Design review of the part shown in the three views and the two pictorial views. Dimensions are in mm from the part's minimum x, y and z. A direction names the side the tool comes from. Round coordinates to 2 decimals unless told otherwise and drop trailing zeros. Loops run counter-clockwise (first coordinate to the right, second up) from the corner with the lowest first, then second, coordinate; pieces in that order, holes last.
1. Consider section A-A on x = 15.53. State the section outline as (y, z) points (1 decimal).
2. Clearance check with flat-ended pins moving along their axes: pin 1 Ø4 at (y, z) = (45.5, 5) entering from -X; pin 2 Ø3 at (y, z) = (77, 1.5) entering from +X; pin 3 Ø7 at (x, y) = (80.482, 66.756) entering from -Z; pin 4 Ø1 at (y, z) = (75.5, 7) entering from +X (1 decimal). State where each tip first meets the part, or that it passes through.
3. To check wall thickness, follow line 1 along Y through (x, z) = (79.5, 5.25) (1 decimal); line 2 along X through (y, z) = (69, 7.5) (1 decimal); line 3 along X through (y, z) = (31.5, 5.75) (1 decimal). State the ranges of each line that lie inside material, in increasing order.
4. Consider section B-B on z = 4.25. State how many separate pieces and enclosed holes the cut face has, then the cut area to 3 significant figures.
5. Tool access review of the marked faces 1 and 2: name each direction out of +Z, -Z, +X, -X, +Y, -Y from which nothing blocks a thin tool from reaching the whole face with its end or side.
6. Draft analysis for pull direction Y (two halves, no side actions). For the marked faces 3, 4 and 5, state which applies: released by +Y, released by -Y, zero draft, split by the parting line, or undercut.
7. Consider section D-D on y = 23.5. State the section outline as (x, z) points (1 decimal).
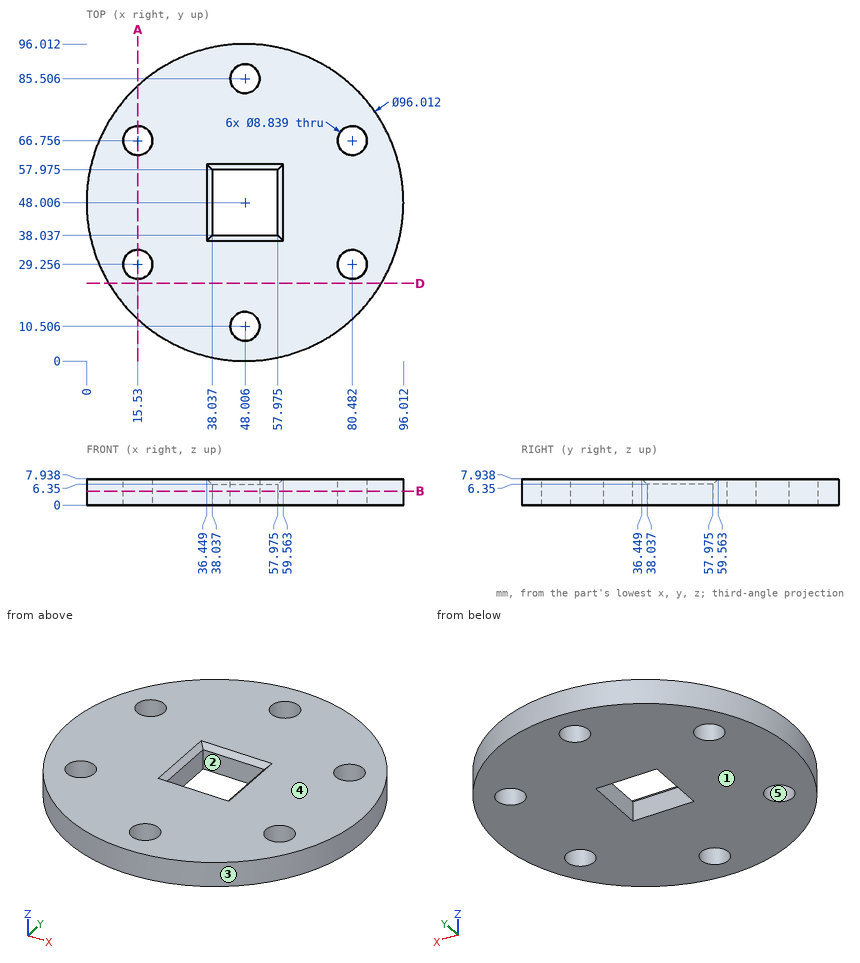
Resolved:
1. outline: (12.7, 0) - (24.8, 0) - (24.8, 7.9) - (12.7, 7.9) - close; (33.7, 0) - (62.3, 0) - (62.3, 7.9) - (33.7, 7.9) - close; (71.2, 0) - (83.4, 0) - (83.4, 7.9) - (71.2, 7.9) - close
2. pin 1: stops at x = 0
2. pin 2: stops at x = 87.36
2. pin 3: passes through
2. pin 4: stops at x = 87.7
3. line 1: y = 11.8 to 24.9, 33.6 to 62.4, 71.1 to 84.2
3. line 2: x = 4.8 to 11.7, 19.3 to 76.7, 84.3 to 91.2
3. line 3: x = 2.9 to 11.7, 19.3 to 76.7, 84.3 to 93.1
4. separate pieces: 1
4. enclosed holes: 7
4. area: 6,470 mm2
5. face 1: -Z, +X, -X, +Y, -Y
5. face 2: +Z, -Z
6. face 3: split by the parting line
6. face 4: zero draft
6. face 5: undercut
7. outline: (6.7, 0) - (89.3, 0) - (89.3, 7.9) - (6.7, 7.9) - close
